Read the model definition and answer for the solid it produces. Units are mm, in the model's axes. A direction names the side the tool comes from. Round coordinates to 2 decimals unless told otherwise and drop trailing zeros. Order: outer loops, then holes, each group sorted by start corner. A loop starts at its lowest first (then second) coordinate and runs counter-clockwise, first axis right, second up. Notation, with made-up numbers: (57.25, 76) - (71.25, 76) arc R25 ccw to (71.25, 109) - close; hole circle Ø8 at (64.25, 51.5). An arc over 180 degrees is marked (long way). Put each result on its own line as item: value. Start each with the question number.
Q1. Section C-C on z = -10.5 is taken. State how many separate pieces and enclosed holes the cut face has, then the cut area to 3 significant figures.
Q2. Which of the six approach directions +Z, -Z, +X, -X, +Y, -Y give full straight-line access (tool end or side, diameter ignored) to faces 1 (the face through (0, 16, -6)), 2 (the face through (-10, -11, -6)), 3 (the face through (-11, 26, -2))?
Q3. Section B-B on x = -17.5 is taken. Give the vertices of the cut face in (y, z).
Q4. For a pull along Z with two mould halves and no side action, classify faces 4 (the face through (7.692, -7.863, -6.409)), 5 (the face through (-46.094, -0.264, -12.494)), 6 (the face through (0, 28, -9)), 7 (the face through (0.2, 30.8, -4)) as pulls with the +Z half, pulls with the -Z half, needs draft (parallel to the pull), parting line crosses it, or undercut.
Q5. Find the intervals of material crossed by line 1 along Y through (x, z) = (0, -10.15); line 2 along Y through (x, z) = (0, -8); line 3 along Y through (x, z) = (-63, -7.5), in increasing order. Write a range as from..to.
Q6. Section D-D on x = -66 is taken. Give the vertices of the cut face in (y, z), then the cut area to 3 significant figures.
Q7. Each of these flat-tipped pins is pushed along its axis until it touches: pin 1 Ø10.5 at (x, y) = (0, 35) entering from +Z; pin 2 Ø3 at (x, y) = (-29, 6) entering from +Z; pin 3 Ø6 at (x, z) = (-40, -11.5) entering from -Y; pin 4 Ø2 at (y, z) = (24.5, -1) entering from -X. Where does it stop, or does it pass through?
Q8. Section A-A on z = -6.5 is taken. Give the vertices of the cut face in (x, y).
Autodesk Inventor part; units mm, degrees
ref_plane "YZ Plane" through (0, 0, 0) normal (1, 0, 0) x (0, 1, 0)
ref_plane "XZ Plane" through (0, 0, 0) normal (0, 1, 0) x (-1, 0, 0)
ref_plane "XY Plane" through (0, 0, 0) normal (0, 0, 1) x (1, 0, 0)
sketch "Boceto1" plane through (0, 0, 0) normal (0, 0, 1) x (1, 0, 0)
  circle A0 centre (0, 0) radius 4
  arc A1 (0, -11) -> (11, 0) centre (0, 0) ccw
  line L0 (0, -11) -> (-21, -11)
  line L1 (0, -11) -> (0, 35) construction
  circle A2 centre (0, 35) radius 4
  arc A3 (11, 35) -> (-11, 35) centre (0, 35) ccw
  line L2 (11, 35) -> (11, 0)
  line L3 (-21, -11) -> (-21, 11)
  line L4 (-21, 11) -> (-16, 11)
  line L5 (0, 35) -> (-11, 35) construction
  line L6 (-11, 35) -> (-11, 16)
  arc A4 (-16, 11) -> (-11, 16) centre (-16, 16) ccw
  dimension "d0" = 8
  dimension "d1" = 22
  dimension "d2" = 21
  dimension "d3" = 46
  dimension "d4" = 8
  dimension "d5" = 22
  dimension "d6" = 22
  dimension "d7" = 5
extrude "Extrusión1" add sketch "Boceto1" against normal blind 13
sketch "Boceto2" plane through (11, 0, 0) normal (1, 0, 0) x (0, 0, -1)
  line L0 (0, 0) -> (4, 0) construction
  line L1 (0, 0) -> (13, 0) construction
  line L2 (0, 35) -> (13, 35)
  line L3 (13, 31) -> (0, 31)
  line L4 (4, 0) -> (9, 0) construction
  line L5 (13, -11) -> (13, 0)
  line L6 (9, 0) -> (13, 0) construction
  line L7 (0, 16) -> (13, 16) construction
  line L8 (4, 16) -> (4, 49.4932)
  line L9 (4, 49.4932) -> (9, 49.4932)
  line L10 (9, 49.4932) -> (9, 16)
  line L11 (4, 16) -> (9, 16)
  line L12 (13, 35) -> (13, 46)
  dimension "d10" = 4
  dimension "d11" = 5
  dimension "d12" = 33.4932
  dimension "d13" = 5
  dimension "d14" = 4
extrude "Extrusión2" cut sketch "Boceto2" against normal through all
sketch "Boceto3" plane through (-21, -11, 0) normal (-1, 0, 0) x (0, 0, 1)
  line L0 (-13, 0) -> (-13, 22)
  circle A0 centre (-6.5, 11) radius 6
  line L1 (0, 22) -> (-13, 22)
  line L2 (-6.5, 22) -> (-6.5, 0) construction
  line L3 (0, 0) -> (-13, 0)
  line L4 (0, 11) -> (-13, 11) construction
  line L5 (-13, 11) -> (0, 11)
  dimension "d26" = 12
extrude "Extrusión3" add sketch "Boceto3" along normal blind 51
thread "Rosca1"
chamfer "Chaflán1" distance 0.1 angle 45 1 edges at (-72, 0, -12.5) measured on face at (-72, -0.4786, -4.5581)
properties part number "19_UnionB"
Findings:
1. separate pieces: 1
1. enclosed holes: 2
1. area: 1,760 mm2
2. face 1: +X, -X, +Y
2. face 2: +Z, -Z, +X, -X, -Y
2. face 3: +Z, -Z, -X, +Y
3. outline: (-11, -13) - (11, -13) - (11, 0) - (-11, 0) - close
4. face 4: needs draft
4. face 5: parting line crosses it
4. face 6: undercut
4. face 7: undercut
5. line 1: -11..-4, 4..31, 39..46
5. line 2: -11..-4, 4..16
5. line 3: -5.92..5.92
6. outline: circle Ø12 at (0, -6.5)
6. area: 113 mm2
7. pin 1: z = 0
7. pin 2: z = -2.53
7. pin 3: y = -5.66
7. pin 4: x = -11
8. outline: (-72, -5.9) - (-71.9, -6) - (-21, -6) - (-21, -11) - (0, -11) arc R11 ccw to (11, 0) - (11, 16) - (-11, 16) arc R5 cw to (-16, 11) - (-21, 11) - (-21, 6) - (-71.9, 6) - (-72, 5.9) - close; hole circle Ø8 at (0, 0)
